from build123d import *

# Parameters (mm, degrees)
BASPROSKE_W         = 3
BASPROSKE_H         = 24.5
TOOTHCUT_DEPTH      = 35.777866525
TEETHCUTS_COUNT     = 26
TEETHCUTS_ANGLE     = 346.153846154
BORSKE_R            = 3
BORE_DEPTH          = 50.0000508
BOSS_EXTRUDE1_START = 3
SKETCH2_R           = 3
BOSS_EXTRUDE1_DEPTH = 3


with BuildPart() as part:
    # BasProSke → Base-Revolve (revolve)
    with BuildSketch(Plane(origin=(0, 0, 0), x_dir=(1, 0, 0), z_dir=(0, 1, 0)), mode=Mode.PRIVATE) as base_revolve_sk:
        with Locations((1.5, 12.25)):
            Rectangle(BASPROSKE_W, BASPROSKE_H)
    revolve(base_revolve_sk.sketch.rotate(Axis((-10, 0, 0), (1, 0, 0)), 180), axis=Axis((-10, 0, 0), (1, 0, 0)))

    # TooCutSke → ToothCut (cut, through all)
    with BuildSketch(Plane(origin=(0, 0, 0), x_dir=(0, 0, -1), z_dir=(1, 0, 0))):
        with BuildLine():
            ThreePointArc((0.813448928, 20.545402967), (0, 20.5615), (-0.813448928, 20.545402967))
            ThreePointArc((-0.813448928, 20.545402967), (-1.408477569, 22.569593712), (-2.4536582, 24.402352481))
            ThreePointArc((-2.4536582, 24.402352481), (0, 24.5254), (2.4536582, 24.402352481))
            ThreePointArc((2.4536582, 24.402352481), (1.408477569, 22.569593712), (0.813448928, 20.545402967))
        make_face()
    toothcut = extrude(amount=TOOTHCUT_DEPTH, mode=Mode.SUBTRACT)

    # TeethCuts: ToothCut ×26 about axis
    teethcuts_axis = Axis((-10, 0, 0), (1, 0, 0))
    for i in range(1, TEETHCUTS_COUNT):
        add(toothcut.rotate(teethcuts_axis, i * TEETHCUTS_ANGLE / (TEETHCUTS_COUNT - 1)), mode=Mode.SUBTRACT)

    # BorSke → Bore (cut, symmetric)
    with BuildSketch(Plane(origin=(0, 0, 0), x_dir=(0, 0, -1), z_dir=(1, 0, 0))):
        with Locations(Location((0, 0, 0), (0, 0, 180))):
            Circle(BORSKE_R)
    extrude(amount=BORE_DEPTH, both=True, mode=Mode.SUBTRACT)

    # Sketch2 → Boss-Extrude1 (add)
    with BuildSketch(Plane(origin=(0, 0, 0), x_dir=(0, 0, -1), z_dir=(1, 0, 0)).offset(BOSS_EXTRUDE1_START)):
        with BuildLine():
            Line((0, -6), (-54, -6))
            ThreePointArc((-54, -6), (-60, 0), (-54, 6))
            Line((-54, 6), (0, 6))
            ThreePointArc((0, 6), (6, 0), (0, -6))
        make_face()
        with Locations((-54, 0)):
            Circle(SKETCH2_R, mode=Mode.SUBTRACT)
        with Locations(Location((0, 0, 0), (0, 0, 180))):
            Circle(SKETCH2_R, mode=Mode.SUBTRACT)
    extrude(amount=-BOSS_EXTRUDE1_DEPTH)


solid = part.part
Could you check a few things on this model? Use its own coordinates, in mm. A direction names the side the tool comes from. Round coordinates to 2 decimals unless told otherwise and drop trailing zeros. Order: outer loops, then holes, each group sorted by start corner. A loop starts at its lowest first (then second) coordinate and runs counter-clockwise, first axis right, second up.
Q1. Imagine slicing it at B-B, the plane x = 1.1. State how many separate pieces and enclosed holes the cut face has, then the cut area to 3 significant figures.
Geometry says:
separate pieces: 1
enclosed holes: 2
area: 1,970 mm2
Q2. Imagine slicing it at A-A, the plane z = 0. List the corners of the cut face in (x, y) for me.
Geometry says:
outline: (0, -20.56) - (3, -20.56) - (3, -3) - (0, -3) - close; (0, 3) - (3, 3) - (3, 20.56) - (0, 20.56) - close
Q3. I'm going to push flat-ended pins straight in: P1, Ø5.5, axis at y = 0, z = 54, coming from the +X side; P2, Ø1.5, axis at x = 1.5, z = 47.5, coming from the -Y side; P3, Ø1.5, axis at x = 1.5, z = 35.5, coming from the +Y side. Where does each tip first touch, or does it pass through?
Geometry says:
P1: passes through
P2: stops at y = -6
P3: stops at y = 6
Q4. Please list where these lines run through material, in increasing order: probe 1 along Y at (x, z) = (1.8, 0); probe 2 along Y at (x, z) = (1.7, 54); probe 3 along Y at (x, z) = (1.8, -17).
Geometry says:
probe 1: y = -20.56 to -3, 3 to 20.56
probe 2: y = -6 to -3, 3 to 6
probe 3: y = -16.36 to -12.93, -11.57 to 11.57, 12.93 to 16.36
Q5. Which directions (+Z, -Z, +X, -X, +Y, -Y) give clear straight access to the entire face, cutting with the end or side of a thin tool? Please do faces 4 (the face through (1.48, -17.79, 13.9)), 5 (the face through (1.5, -4.1, -22.2)), 6 (the face through (1.5, -19.3, -11.7)).
Geometry says:
face 4: +X, -X
face 5: -Z, +X, -X
face 6: +X, -X, -Y
Q6. Imagine slicing it at D-D, the plane z = 26.5. List the corners of the cut face in (x, y) for me, then the cut area to 3 significant figures.
Geometry says:
outline: (0, -6) - (3, -6) - (3, 6) - (0, 6) - close
area: 36.0 mm2
Q7. Thinking about a two-plate mould opening in Y: for faces 1 (the face through (1.48, -13.94, 17.75)), 2 (the face through (1.48, -21.54, -6.74)), 3 (the face through (2, 0, 60)), which applies, released by +Y, released by -Y, zero draft, split by the parting line, or undercut?
Geometry says:
face 1: undercut
face 2: released by -Y
face 3: split by the parting line
Q8. Imagine slicing it at C-C, the plane z = 53. List the corners of the cut face in (x, y) for me, then the cut area to 3 significant figures.
Geometry says:
outline: (0, -6) - (3, -6) - (3, -2.83) - (0, -2.83) - close; (0, 2.83) - (3, 2.83) - (3, 6) - (0, 6) - close
area: 19.0 mm2
